```python
from build123d import *

# Parameters (mm, degrees)
F1_DEPTH = 6.35
F2_SIZE  = 2.54


with BuildPart() as f1:
    # F0 (on Top) → F1 (new body)
    with BuildSketch(Plane.XY):
        with BuildLine():
            ThreePointArc((-4.7385636703, 21.2063813699), (-7.7641105007, 22.0872871715), (-10.6362471428, 23.3837283631))
            Line((-10.6362471428, 23.3837283631), (-16.6063122451, 4.8134931872))
            Line((-16.6063122451, 4.8134931872), (-16.6063122451, -97.1717238426))
            Line((-16.6063122451, -97.1717238426), (-4.7385636703, 21.2063813699))
        make_face()
        with BuildLine():
            Line((16.6063122451, 4.8134931872), (10.6362471428, 23.3837283631))
            ThreePointArc((10.6362471428, 23.3837283631), (7.7641105007, 22.0872871715), (4.7385636703, 21.2063813699))
            Line((4.7385636703, 21.2063813699), (16.6063122451, -97.1717238426))
            Line((16.6063122451, -97.1717238426), (16.6063122451, 4.8134931872))
        make_face()
        with BuildLine():
            ThreePointArc((4.7385636703, 21.2063813699), (7.7641105007, 22.0872871715), (10.6362471428, 23.3837283631))
            Line((10.6362471428, 23.3837283631), (9.584756598, 26.6544509379))
            ThreePointArc((9.584756598, 26.6544509379), (7.0687284773, 25.427604555), (4.4000770701, 24.5827085745))
            Line((4.4000770701, 24.5827085745), (4.7385636703, 21.2063813699))
        make_face()
        with BuildLine():
            ThreePointArc((4.4000770701, 24.5827085745), (7.0687284773, 25.427604555), (9.584756598, 26.6544509379))
            Line((9.584756598, 26.6544509379), (6.36176439, 36.6797558963))
            ThreePointArc((6.36176439, 36.6797558963), (4.9698835047, 35.5533311125), (3.3834871789, 34.7229625859))
            Line((3.3834871789, 34.7229625859), (4.4000770701, 24.5827085745))
        make_face()
        with BuildLine():
            Line((-9.584756598, 26.6544509379), (-10.6362471428, 23.3837283631))
            ThreePointArc((-10.6362471428, 23.3837283631), (-7.7641105007, 22.0872871715), (-4.7385636703, 21.2063813699))
            Line((-4.7385636703, 21.2063813699), (-4.4000770701, 24.5827085745))
            ThreePointArc((-4.4000770701, 24.5827085745), (-7.0687284773, 25.427604555), (-9.584756598, 26.6544509379))
        make_face()
        with BuildLine():
            Line((-6.36176439, 36.6797558963), (-9.584756598, 26.6544509379))
            ThreePointArc((-9.584756598, 26.6544509379), (-7.0687284773, 25.427604555), (-4.4000770701, 24.5827085745))
            Line((-4.4000770701, 24.5827085745), (-3.3834871789, 34.7229625859))
            ThreePointArc((-3.3834871789, 34.7229625859), (-4.9698835047, 35.5533311125), (-6.36176439, 36.6797558963))
        make_face()
        with BuildLine():
            ThreePointArc((10.6362471428, 23.3837283631), (19.2483201468, 31.6259749482), (22.417739409, 43.1175897928))
            ThreePointArc((22.417739409, 43.1175897928), (-11.4916148446, 62.3659099396), (-10.6362471428, 23.3837283631))
            Line((-10.6362471428, 23.3837283631), (-9.584756598, 26.6544509379))
            ThreePointArc((-9.584756598, 26.6544509379), (-9.4950746919, 59.6326149698), (19.05, 43.1175897928))
            ThreePointArc((19.05, 43.1175897928), (16.515025177, 33.622515101), (9.584756598, 26.6544509379))
            Line((9.584756598, 26.6544509379), (10.6362471428, 23.3837283631))
        make_face()
        with BuildLine():
            ThreePointArc((9.0508425814, 43.1175897928), (-3.4884397228, 51.4691489127), (-6.36176439, 36.6797558963))
            ThreePointArc((-6.36176439, 36.6797558963), (-4.9698835047, 35.5533311125), (-3.3834871789, 34.7229625859))
            Line((-3.3834871789, 34.7229625859), (-1.8990624038, 38.405906231))
            ThreePointArc((-1.8990624038, 38.405906231), (-2.8424604649, 47.3279126433), (5.08, 43.1175897928))
            ThreePointArc((5.08, 43.1175897928), (4.2103228505, 40.2751293279), (1.8990624038, 38.405906231))
            Line((1.8990624038, 38.405906231), (3.3834871789, 34.7229625859))
            ThreePointArc((3.3834871789, 34.7229625859), (4.9698835047, 35.5533311125), (6.36176439, 36.6797558963))
            ThreePointArc((6.36176439, 36.6797558963), (8.3515591199, 39.62915007), (9.0508425814, 43.1175897928))
        make_face()
    extrude(amount=F1_DEPTH)

    # F2
    f2_edges = [f1.edges().sort_by_distance(p)[0] for p in [
        (-16.606312, -46.179115, 6.35),
        (16.606312, -46.179115, 6.35),
        (16.606312, -46.179115, 0),
        (-16.606312, -46.179115, 0),
    ]]
    chamfer(f2_edges, length=F2_SIZE)


solid = f1.part
```
Can you work these out from the model? Positions are in its coordinate system, mm. A direction names the side the tool comes from. Coordinates: 2 decimals unless noted, no trailing zeros. Order: outer loops, then holes, each group sorted by start corner. A loop starts at its lowest first (then second) coordinate and runs counter-clockwise, first axis right, second up.
1. If we section it at B-B (y = 40): Please give me the cut outline in (x, z), then the cut area to 3 significant figures.
2. Thinking about a two-plate mould opening in Y: for faces 1 (the face through (13, 16.03, 3.13)), 2 (the face through (-7, 12, 6.35)), 3 (the face through (-2.65, 36.54, 3.13)), which applies, +Y half, -Y half, draft (parallel to the pull), parting line (faces both ways), or undercut?
3. If we section it at D-D (y = -55.5): Please give me the cut outline in (x, z).
4. For faces 4 (the face through (15.319, -42.998, 1.252)), 5 (the face through (7.996, 31.597, 3.131)), 6 (the face through (2.63, 36.59, 3.13)), 7 (the face through (-12.916, 16.292, 3.131)), which set-ups out of +Z, -Z, +X, -X, +Y, -Y let a thin tool reach every point of the face, with its end or its side?
5. I need wall thicknesses on line 1 (X direction, y = 43.5, z = 2.75); line 2 (X direction, y = 30.5, z = 2); line 3 (Y direction, x = 0, z = 5). Which ranges of each line are inside material? Lowest first, please.
6. If we section it at A-A (x = 0): Please give me the cut outline in (y, z).
7. I'm going to push flat-ended pins straight in: pin 1 (3 mm diameter, centred on y = 2.5, z = 5, fed in from -X); pin 2 (1 mm diameter, centred on x = -1.5, z = 2.5, fed in from -Y); pin 3 (6 mm diameter, centred on x = -17.5, y = -63, fed in from -Z). Where does each tip first touch, or does it pass through?
8. If we section it at C-C (z = 1.25): Please give me the cut outline in (x, y), then the cut area to 3 significant figures.
Entries:
1. outline: (-22.2, 0) - (-18.79, 0) - (-18.79, 6.35) - (-22.2, 6.35) - close; (-8.5, 0) - (-4.01, 0) - (-4.01, 6.35) - (-8.5, 6.35) - close; (4.01, 0) - (8.5, 0) - (8.5, 6.35) - (4.01, 6.35) - close; (18.79, 0) - (22.2, 0) - (22.2, 6.35) - (18.79, 6.35) - close
1. area: 100 mm2
2. face 1: undercut
2. face 2: draft
2. face 3: -Y half
3. outline: (-16.61, 2.54) - (-14.07, 0) - (-12.43, 0) - (-12.43, 6.35) - (-14.07, 6.35) - (-16.61, 3.81) - close; (12.43, 0) - (14.07, 0) - (16.61, 2.54) - (16.61, 3.81) - (14.07, 6.35) - (12.43, 6.35) - close
4. face 4: -Z, +X, -Y
4. face 5: +Z, -Z
4. face 6: +Z, -Z, -Y
4. face 7: +Z, -Z, -X
5. line 1: x = -22.41 to -19.05, -9.04 to -5.07, 5.07 to 9.04, 19.05 to 22.41
5. line 2: x = -18.53 to -14.27, -8.35 to -3.81, 3.81 to 8.35, 14.27 to 18.53
5. line 3: y = 48.2 to 52.17, 62.17 to 65.54
6. outline: (48.2, 0) - (52.17, 0) - (52.17, 6.35) - (48.2, 6.35) - close; (62.17, 0) - (65.54, 0) - (65.54, 6.35) - (62.17, 6.35) - close
7. pin 1: stops at x = -16.61
7. pin 2: stops at y = 38.16
7. pin 3: stops at z = 0.43
8. outline: (-15.32, -84.3) - (-3.38, 34.72) - (-1.9, 38.41) arc R5.08 cw (long way) to (1.9, 38.41) - (3.38, 34.72) - (15.32, -84.3) - (15.32, 8.83) - (10.64, 23.38) arc R22.42 ccw (long way) to (-10.64, 23.38) - (-15.32, 8.83) - close; hole (-9.58, 26.65) - (-6.36, 36.68) arc R9.05 cw (long way) to (6.36, 36.68) - (9.58, 26.65) arc R19.05 ccw (long way) to start
8. area: 1,730 mm2
